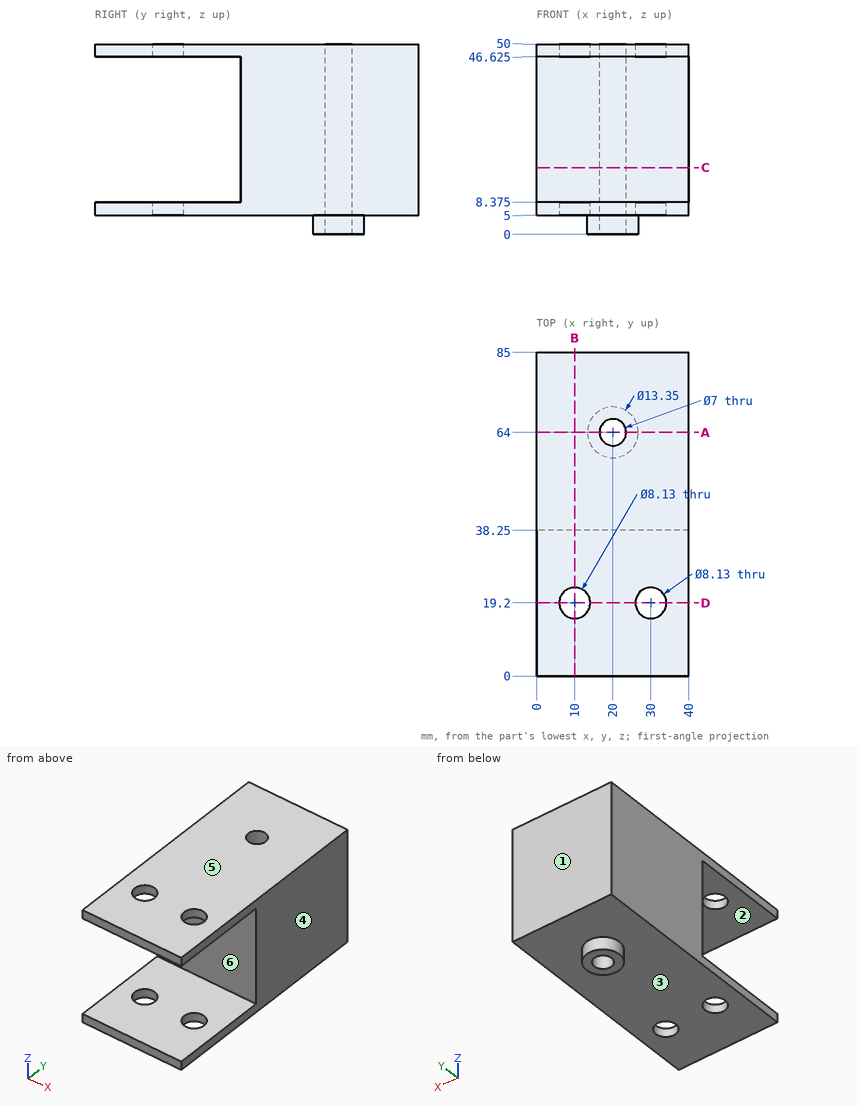
Geometry check sheet. Reference: drawing and pictorial views, mm from the part's lowest x, y, z. A direction names the side the tool comes from. Round coordinates to 2 decimals unless told otherwise and drop trailing zeros. Order: outer loops, then holes, each group sorted by start corner. A loop starts at its lowest first (then second) coordinate and runs counter-clockwise, first axis right, second up. Notation, with made-up numbers: M 82,83.25 L 138,83.25 A9 ccw 138,93.25 Z; hole C -14.5,-8.5 d9. An arc over 180 degrees is marked long. Write item = value, one per line.
Q1. Depth check by flat-ended pin: pin 1 Ø1.5 at (x, z) = (20, 40) entering from -Y; pin 2 Ø19 at (x, y) = (26, 19) entering from -Z. Enter the tip coordinate at first touch or a pass-through.
Answer block:
pin_1 = 38.25
pin_2 = 5
Q2. Section check B-B (x = 10). Enter the section's corners in (y, z) (3 decimals).
Answer block:
outline = M 0,5 L 15.135,5 L 15.135,8.375 L 0,8.375 Z; M 0,46.625 L 15.135,46.625 L 15.135,50 L 0,50 Z; M 23.265,5 L 85,5 L 85,50 L 23.265,50 L 23.265,46.625 L 38.25,46.625 L 38.25,8.375 L 23.265,8.375 Z
Q3. Set-up check for the marked faces 1 and 2: record each of +Z, -Z, +X, -X, +Y, -Y from which the full face is reachable in a straight line by a thin tool's end or side.
Answer block:
face_1 = +Z, -Z, +X, -X, +Y
face_2 = +X, -X, -Y
Q4. Section check C-C (z = 17.5). Enter the section's corners in (x, y).
Answer block:
outline = M 0,38.25 L 40,38.25 L 40,85 L 0,85 Z; hole C 20,64 d7
Q5. Section check D-D (y = 19.2). Enter the section's corners in (x, z) (3 decimals), plus the area to 3 significant figures.
Answer block:
outline = M 0,5 L 5.935,5 L 5.935,8.375 L 0,8.375 Z; M 0,46.625 L 5.935,46.625 L 5.935,50 L 0,50 Z; M 14.065,5 L 25.935,5 L 25.935,8.375 L 14.065,8.375 Z; M 14.065,46.625 L 25.935,46.625 L 25.935,50 L 14.065,50 Z; M 34.065,5 L 40,5 L 40,8.375 L 34.065,8.375 Z; M 34.065,46.625 L 40,46.625 L 40,50 L 34.065,50 Z
area = 160 mm^2
Q6. Section check A-A (y = 64). Enter the section's corners in (x, z) (3 decimals), plus the area to 3 significant figures.
Answer block:
outline = M 0,5 L 13.325,5 L 13.325,0 L 16.5,0 L 16.5,50 L 0,50 Z; M 23.5,0 L 26.675,0 L 26.675,5 L 40,5 L 40,50 L 23.5,50 Z
area = 1,520 mm^2
Q7. Release check for a two-part mould opening along Z. For the marked faces 3, 4, 5 and 6 record: released by +Z, released by -Z, zero draft, split by the parting line, or undercut.
Answer block:
face_3 = released by -Z
face_4 = zero draft
face_5 = released by +Z
face_6 = undercut
Q8. Scan lines: line 1 (X direction, y = 19, z = 48); line 2 (Z direction, x = 18, y = 31) (3 decimals); line 3 (Y direction, x = 10, z = 6.85) (3 decimals). Record each from-to range of solid material in increasing order.
Answer block:
line_1 = 0 to 5.94, 14.06 to 25.94, 34.06 to 40
line_2 = 5 to 8.375, 46.625 to 50
line_3 = 0 to 15.135, 23.265 to 85
